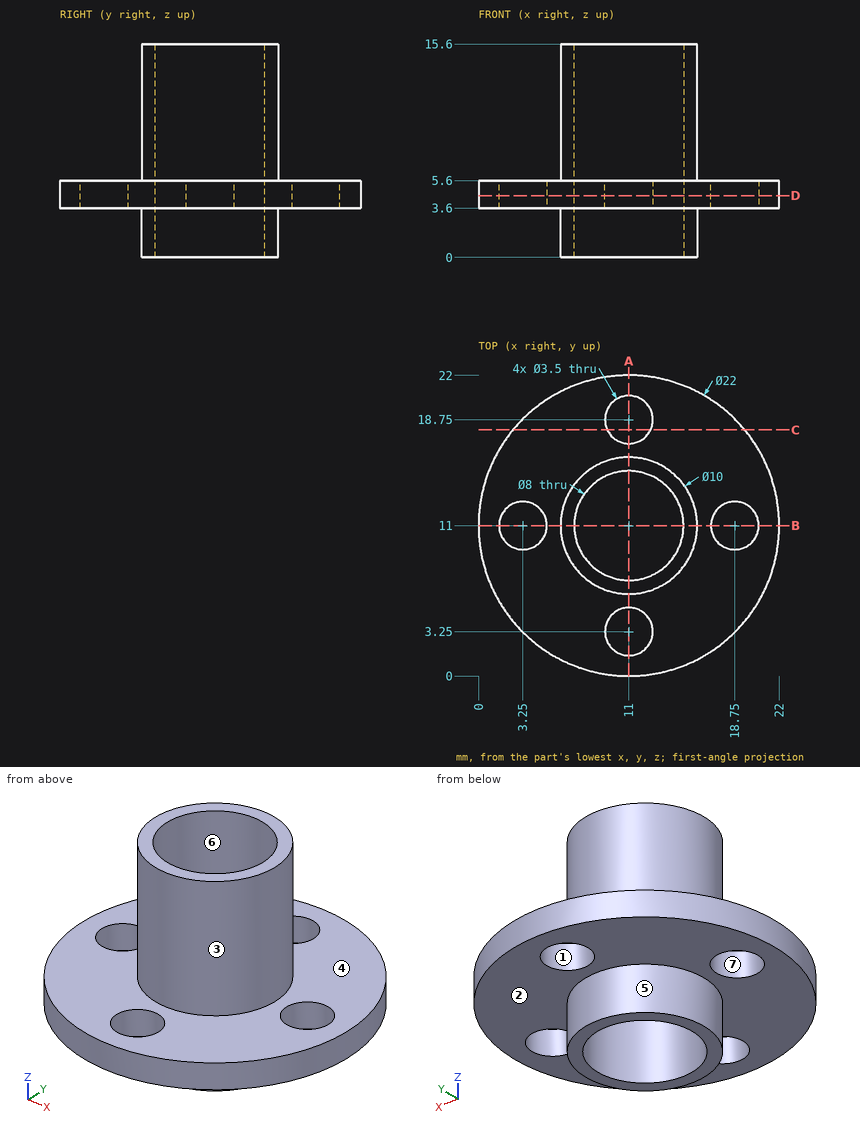
The drawing under review shows one solid part. Ordinate dimensions are in mm from its lowest x, y, z. A direction names the side the tool comes from. Give positions to 0.01 mm unless a question says otherwise; leave off trailing zeros. Order: outer loops, then holes, each group sorted by start corner. A loop starts at its lowest first (then second) coordinate and runs counter-clockwise, first axis right, second up. Notation, with made-up numbers: (-15, -36) -> (16, -36) arc R27 cw to (16, -11) -> close; hole circle Ø9 at (62.5, 9). An arc over 180 degrees is marked (long way). Write item = value, one per line.
1) Draft analysis for pull direction X (two halves, no side actions). For the marked faces 4, 5, 6 and 7, state which applies: pulls with the +X half, pulls with the -X half, needs draft (parallel to the pull), parting line crosses it, or undercut.
Findings:
face_4 = needs draft
face_5 = parting line crosses it
face_6 = undercut
face_7 = undercut
2) We need section A-A, the plane x = 11. Give the boundary of the cut face in (y, z).
Findings:
outline = (0, 3.6) -> (1.5, 3.6) -> (1.5, 5.6) -> (0, 5.6) -> close; (5, 3.6) -> (6, 3.6) -> (6, 0) -> (7, 0) -> (7, 15.6) -> (6, 15.6) -> (6, 5.6) -> (5, 5.6) -> close; (15, 0) -> (16, 0) -> (16, 3.6) -> (17, 3.6) -> (17, 5.6) -> (16, 5.6) -> (16, 15.6) -> (15, 15.6) -> close; (20.5, 3.6) -> (22, 3.6) -> (22, 5.6) -> (20.5, 5.6) -> close
3) Insertion check: pin 1 (4 mm diameter, centred on x = 19.5, z = 2, fed in from -Y); pin 2 (6 mm diameter, centred on x = 18, y = 7, fed in from -Z); pin 3 (2 mm diameter, centred on y = 13, z = 11, fed in from -X). Each pin has a flat end and moves straight along its axis. Give the tip position at first contact, or say it passes through.
Findings:
pin_1 = 2.77
pin_2 = 3.6
pin_3 = 6.1
4) To check wall thickness, follow L1, parallel to Y at x = 11, z = 4.7; L2, parallel to Y at x = 11, z = 11; L3, parallel to Z at x = 19.5, y = 17. State the ranges of each line that lie inside material, in increasing order. Write a range as from..to.
Findings:
L1 = 0..1.5, 5..7, 15..17, 20.5..22
L2 = 6..7, 15..16
L3 = 3.6..5.6
5) We need section D-D, the plane z = 4.5. Give the boundary of the cut face in (x, y), and give its area (3 significant figures).
Findings:
outline = circle Ø22 at (11, 11); hole circle Ø3.5 at (3.25, 11); hole circle Ø8 at (11, 11); hole circle Ø3.5 at (11, 3.25); hole circle Ø3.5 at (11, 18.75); hole circle Ø3.5 at (18.75, 11)
area = 291 mm^2
6) For the marked faces 1, 2 and 3, list the 3-axis set-ups (+Z, -Z, +X, -X, +Y, -Y) from which the entire face can be reached by the end or side of a thin tool; tool diameter is ignored.
Findings:
face_1 = +Z, -Z
face_2 = -Z
face_3 = +Z
7) We need section C-C, the plane y = 18. Give the boundary of the cut face in (x, z).
Findings:
outline = (2.51, 3.6) -> (9.42, 3.6) -> (9.42, 5.6) -> (2.51, 5.6) -> close; (12.58, 3.6) -> (19.49, 3.6) -> (19.49, 5.6) -> (12.58, 5.6) -> close
